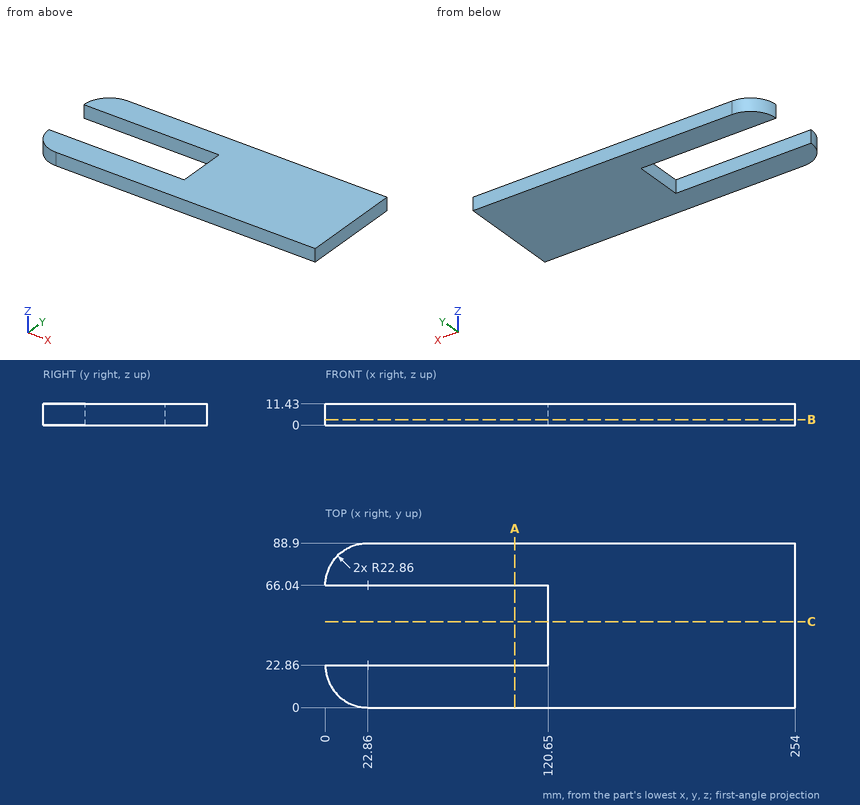
The figure shows three views and two pictorial views of one solid part (mm, origin at its lowest corner). Answer the questions. Give positions to 0.01 mm unless a question says otherwise; leave off trailing zeros. Write each loop counter-clockwise with the first axis right and the second up, starting at its lowest first coordinate (ties: lowest second). Pieces come first, ordered by that corner, then holes. Notation, with made-up numbers: (7, -29.5) -> (55, -29.5) arc R32 cw to (55, 1.5) -> close; hole circle Ø10 at (-7, -0.5). An arc over 180 degrees is marked (long way). Answer as a JSON object with one key per item and string values.
1) Straight lines are drawn through the part: probe 1 along Y at (x, z) = (80.5, 5.5); probe 2 along X at (y, z) = (57, 1.75); probe 3 along X at (y, z) = (83, 4.5). For each, find the intervals that lie inside material, in ascending order. Write a range as from..to.
Findings below:
{"probe 1": "y = 0..22.86, 66.04..88.9", "probe 2": "x = 120.65..254", "probe 3": "x = 7.53..254"}
2) Section B-B on z = 3 is taken. Write down the section's boundary in (x, y).
Findings below:
{"outline": "(0, 22.86) arc R22.86 ccw to (22.86, 0) -> (254, 0) -> (254, 88.9) -> (22.86, 88.9) arc R22.86 ccw to (0, 66.04) -> (120.65, 66.04) -> (120.65, 22.86) -> close"}
3) Flat-ended cylindrical pins translate along their axes: pin 1 Ø1 at (x, y) = (223.5, 27.5) entering from -Z; pin 2 Ø3 at (y, z) = (46.5, 2.5) entering from -X. Find the tip coordinate at first contact, or state that the pin passes through.
Findings below:
{"pin 1": "stops at z = 0", "pin 2": "stops at x = 120.65"}
4) Section C-C on y = 46.5 is taken. Write down the section's boundary in (x, z), then the cut area to 3 significant figures.
Findings below:
{"outline": "(120.65, 0) -> (254, 0) -> (254, 11.43) -> (120.65, 11.43) -> close", "area": "1,520 mm^2"}
5) Section A-A on x = 102.5 is taken. Write down the section's boundary in (y, z), then the cut area to 3 significant figures.
Findings below:
{"outline": "(0, 0) -> (22.86, 0) -> (22.86, 11.43) -> (0, 11.43) -> close; (66.04, 0) -> (88.9, 0) -> (88.9, 11.43) -> (66.04, 11.43) -> close", "area": "523 mm^2"}
